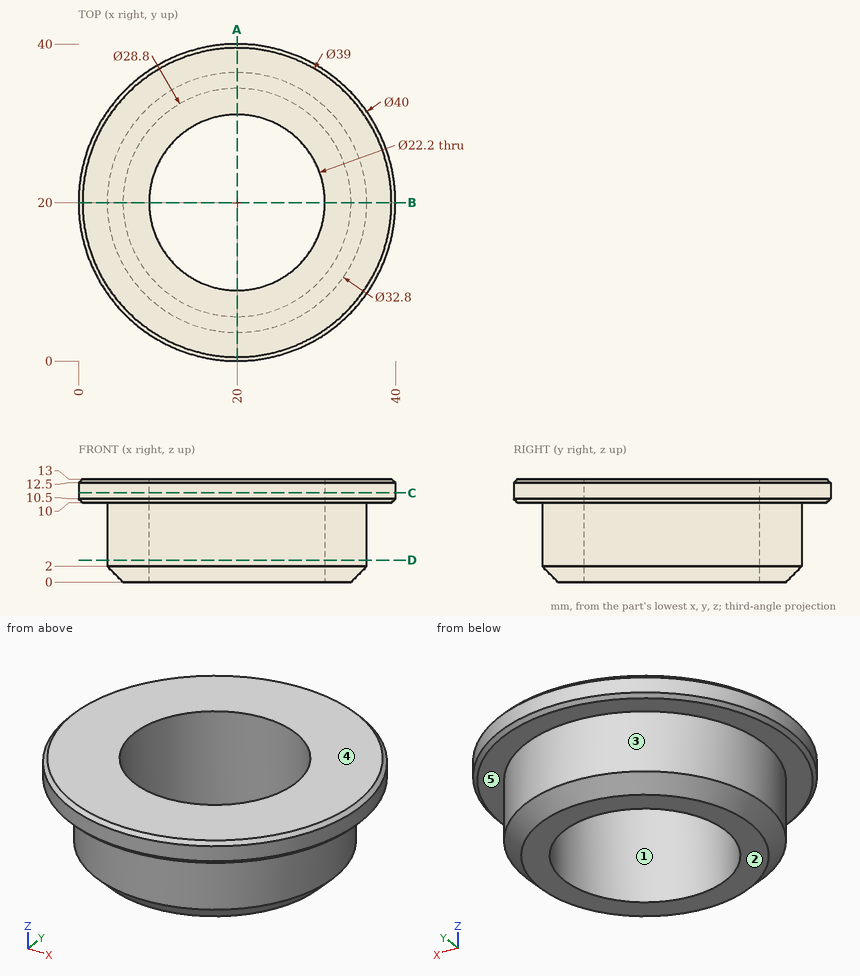
Study the drawing (mm; zero at the part's minimum x, y, z) and answer. A direction names the side the tool comes from. Coordinates: 2 decimals unless noted, no trailing zeros. Order: outer loops, then holes, each group sorted by start corner. A loop starts at its lowest first (then second) coordinate and runs counter-clockwise, first axis right, second up. Notation, with made-up numbers: (55, -14) -> (110, -14) arc R25 cw to (110, 4) -> close; hole circle Ø11 at (85.5, 60). An arc over 180 degrees is marked (long way). Answer in a Markdown table with one row per item. Add a question column.
Item 1: Determine the mould class of the marked faces 1, 2 and 3 for opening direction X: +X half, -X half, draft (parallel to the pull), parting line (faces both ways), or undercut.
Item 2: Find section D-D (z = 2.75). Write down the section's boundary in (x, y), then the cut area to 3 significant figures.
Item 3: Find section A-A (x = 20). Write down the section's boundary in (y, z), then the cut area to 3 significant figures.
Item 4: Each of these flat-tipped pins is pushed along its axis until it touches: P1, Ø3, axis at y = 28.5, z = 3, coming from the -X side; P2, Ø2, axis at y = 22.5, z = 5.5, coming from the +X side; P3, Ø6, axis at x = 36, z = 1.5, coming from the -Y side; P4, Ø4, axis at x = 23.5, y = 4.5, coming from the -Z side. Where does it stop, or does it pass through?
Item 5: Find section C-C (z = 11.25). Write down the section's boundary in (x, y), then the cut area to 3 significant figures.
Item 6: Which of the six approach directions +Z, -Z, +X, -X, +Y, -Y give full straight-line access (tool end or side, diameter ignored) to the marked faces 4 and 5?
Item 7: Find the intervals of material crossed by L1, parallel to Y at x = 20, z = 4; L2, parallel to Y at x = 19, z = 10.25; L3, parallel to X at y = 30, z = 3, in increasing order. Write a range as from..to.
Result set:
| question | item | result |
|---|---|---|
| 1 | face 1 | undercut |
| 1 | face 2 | draft |
| 1 | face 3 | parting line |
| 2 | outline | circle Ø32.8 at (20, 20); hole circle Ø22.2 at (20, 20) |
| 2 | area | 458 mm² |
| 3 | outline | (0, 10.5) -> (0.5, 10) -> (3.6, 10) -> (3.6, 2) -> (5.6, 0) -> (8.9, 0) -> (8.9, 13) -> (0.5, 13) -> (0, 12.5) -> close; (31.1, 0) -> (34.4, 0) -> (36.4, 2) -> (36.4, 10) -> (39.5, 10) -> (40, 10.5) -> (40, 12.5) -> (39.5, 13) -> (31.1, 13) -> close |
| 3 | area | 155 mm² |
| 4 | P1 | stops at x = 5.17 |
| 4 | P2 | stops at x = 36.33 |
| 4 | P3 | stops at y = 10.06 |
| 4 | P4 | stops at z = 0 |
| 5 | outline | circle Ø40 at (20, 20); hole circle Ø22.2 at (20, 20) |
| 5 | area | 870 mm² |
| 6 | face 4 | +Z, +X, -X, +Y, -Y |
| 6 | face 5 | -Z |
| 7 | L1 | y = 3.6..8.9, 31.1..36.4 |
| 7 | L2 | y = 0.28..8.95, 31.05..39.72 |
| 7 | L3 | x = 7..15.18, 24.82..33 |
